Source: CAD feature listing. Evaluate the final solid. Frame: model axes, mm. A direction names the side the tool comes from. Give positions to 0.01 mm unless a question says otherwise; leave off trailing zeros. Order: outer loops, then holes, each group sorted by start corner. A loop starts at its lowest first (then second) coordinate and runs counter-clockwise, first axis right, second up. Notation, with made-up numbers: (76.5, 44) -> (133.5, 44) arc R16 ccw to (133.5, 74) -> close; hole circle Ø6 at (29.5, -8). An arc over 180 degrees is marked (long way). Answer in a Markdown table with one row per item.
```python
from build123d import *

# Parameters (mm, degrees)
F0_W         = 80
F0_H         = 60
F0_W_2       = 72
F0_H_2       = 52
F0_R         = 3
F0_R_2       = 2
F1_DEPTH     = 4
F2_DEPTH     = 30
F3_DEPTH     = 16
F5_R         = 12
F6_R         = 15
F7_S5_R      = 12
F7_T6_DEPTH  = 15
F7_S11_R     = 12
F7_T12_DEPTH = 15
F7_S17_R     = 12
F7_T18_DEPTH = 15
F7_S23_R     = 12
F7_T24_DEPTH = 15


# Not quite as in the source:
# - a fillet or chamfer that OpenCascade refuses, or shapes differently, is made with other operations: its cross-section is extruded or revolved along the edge and cut away or added


with BuildPart() as f1:
    # F0 (on Top) → F1 (new body)
    with BuildSketch(Plane.XY):
        Rectangle(F0_W, F0_H)
        Rectangle(F0_W_2, F0_H_2, mode=Mode.SUBTRACT)
        Rectangle(F0_W_2, F0_H_2)
        with Locations((-30, -20)):
            Circle(F0_R, mode=Mode.SUBTRACT)
        with Locations((30, -20)):
            Circle(F0_R, mode=Mode.SUBTRACT)
        with Locations((-30, 20)):
            Circle(F0_R, mode=Mode.SUBTRACT)
        with Locations((30, 20)):
            Circle(F0_R, mode=Mode.SUBTRACT)
        with Locations((-30, 20)):
            Circle(F0_R)
        with Locations((-30, 20)):
            Circle(F0_R_2, mode=Mode.SUBTRACT)
        with Locations((30, 20)):
            Circle(F0_R)
        with Locations((30, 20)):
            Circle(F0_R_2, mode=Mode.SUBTRACT)
        with Locations((30, -20)):
            Circle(F0_R)
        with Locations((30, -20)):
            Circle(F0_R_2, mode=Mode.SUBTRACT)
        with Locations((-30, -20)):
            Circle(F0_R)
        with Locations((-30, -20)):
            Circle(F0_R_2, mode=Mode.SUBTRACT)
    extrude(amount=F1_DEPTH)

    # F0 (on Top) → F2 (join)
    with BuildSketch(Plane.XY):
        Rectangle(F0_W, F0_H)
        Rectangle(F0_W_2, F0_H_2, mode=Mode.SUBTRACT)
    extrude(amount=F2_DEPTH)

    # F0 (on Top) → F3 (join)
    with BuildSketch(Plane.XY):
        with Locations((-30, 20)):
            Circle(F0_R)
        with Locations((-30, 20)):
            Circle(F0_R_2, mode=Mode.SUBTRACT)
        with Locations((-30, -20)):
            Circle(F0_R)
        with Locations((-30, -20)):
            Circle(F0_R_2, mode=Mode.SUBTRACT)
        with Locations((30, 20)):
            Circle(F0_R)
        with Locations((30, 20)):
            Circle(F0_R_2, mode=Mode.SUBTRACT)
        with Locations((30, -20)):
            Circle(F0_R)
        with Locations((30, -20)):
            Circle(F0_R_2, mode=Mode.SUBTRACT)
    extrude(amount=F3_DEPTH)

    # F4: union 

    # F5
    f5_edges = [f1.edges().sort_by_distance(p)[0] for p in [
        (-36, 26, 17),
        (36, 26, 17),
        (-36, -26, 17),
        (36, -26, 17),
    ]]
    fillet(f5_edges, radius=F5_R)

    # F6
    f6_edges = [f1.edges().sort_by_distance(p)[0] for p in [
        (40, -30, 15),
        (-40, -30, 15),
        (40, 30, 15),
        (-40, 30, 15),
    ]]
    fillet(f6_edges, radius=F6_R)

    # F7: fillet of radius 5.5 on 4 edges, made by hand


with BuildPart() as f7_tool2:
    # F7_s3 → F7_t4 (revolve)
    with BuildSketch(Plane.XZ.offset(-20)):
        with BuildLine():
            ThreePointArc((-21.4990343146, 3.9996), (-25.3890872965, 5.6109127035), (-27.0004, 9.5009656854))
            Line((-27.0004, 9.5009656854), (-27.5505365685, 9.5009656854))
            ThreePointArc((-27.5505365685, 9.5009656854), (-27.5501365685, 6.7504828427), (-27.5501365685, 4))
            Line((-27.5501365685, 4), (-27, 3.4498634315))
            ThreePointArc((-27, 3.4498634315), (-24.2495171573, 3.4498634315), (-21.4990343146, 3.4494634315))
            Line((-21.4990343146, 3.4494634315), (-21.4990343146, 3.9996))
        make_face()
    revolve(axis=Axis((-30, 20, 4), (0, 0, -1)))

    # F7_s5 → F7_t6 (intersect, symmetric)
    with BuildSketch(Plane.XY.offset(8.4)):
        with Locations((-24, 14)):
            Circle(F7_S5_R)
    extrude(amount=F7_T6_DEPTH, both=True, mode=Mode.INTERSECT)


with BuildPart() as f1_1:
    add(f1.part)

    # F7_t1: union F7_tool2
    add(f7_tool2.part)


with BuildPart() as f7_tool8:
    # F7_s9 → F7_t10 (revolve)
    with BuildSketch(Plane.XZ.offset(20)):
        with BuildLine():
            ThreePointArc((-21.4990343146, 3.9996), (-25.3890872965, 5.6109127035), (-27.0004, 9.5009656854))
            Line((-27.0004, 9.5009656854), (-27.5505365685, 9.5009656854))
            ThreePointArc((-27.5505365685, 9.5009656854), (-27.5501365685, 6.7504828427), (-27.5501365685, 4))
            Line((-27.5501365685, 4), (-27, 3.4498634315))
            ThreePointArc((-27, 3.4498634315), (-24.2495171573, 3.4498634315), (-21.4990343146, 3.4494634315))
            Line((-21.4990343146, 3.4494634315), (-21.4990343146, 3.9996))
        make_face()
    revolve(axis=Axis((-30, -20, 4), (0, 0, -1)))

    # F7_s11 → F7_t12 (intersect, symmetric)
    with BuildSketch(Plane.XY.offset(8.4)):
        with Locations((-24, -14)):
            Circle(F7_S11_R)
    extrude(amount=F7_T12_DEPTH, both=True, mode=Mode.INTERSECT)


with BuildPart() as f1_2:
    add(f1_1.part)

    # F7_t7: union F7_tool8
    add(f7_tool8.part)


with BuildPart() as f7_tool14:
    # F7_s15 → F7_t16 (revolve)
    with BuildSketch(Plane.XZ.offset(-20)):
        with BuildLine():
            ThreePointArc((38.5009656854, 3.9996), (34.6109127035, 5.6109127035), (32.9996, 9.5009656854))
            Line((32.9996, 9.5009656854), (32.4494634315, 9.5009656854))
            ThreePointArc((32.4494634315, 9.5009656854), (32.4498634315, 6.7504828427), (32.4498634315, 4))
            Line((32.4498634315, 4), (33, 3.4498634315))
            ThreePointArc((33, 3.4498634315), (35.7504828427, 3.4498634315), (38.5009656854, 3.4494634315))
            Line((38.5009656854, 3.4494634315), (38.5009656854, 3.9996))
        make_face()
    revolve(axis=Axis((30, 20, 4), (0, 0, -1)))

    # F7_s17 → F7_t18 (intersect, symmetric)
    with BuildSketch(Plane.XY.offset(8.4)):
        with Locations((24, 14)):
            Circle(F7_S17_R)
    extrude(amount=F7_T18_DEPTH, both=True, mode=Mode.INTERSECT)


with BuildPart() as f1_3:
    add(f1_2.part)

    # F7_t13: union F7_tool14
    add(f7_tool14.part)


with BuildPart() as f7_tool20:
    # F7_s21 → F7_t22 (revolve)
    with BuildSketch(Plane.XZ.offset(20)):
        with BuildLine():
            ThreePointArc((38.5009656854, 3.9996), (34.6109127035, 5.6109127035), (32.9996, 9.5009656854))
            Line((32.9996, 9.5009656854), (32.4494634315, 9.5009656854))
            ThreePointArc((32.4494634315, 9.5009656854), (32.4498634315, 6.7504828427), (32.4498634315, 4))
            Line((32.4498634315, 4), (33, 3.4498634315))
            ThreePointArc((33, 3.4498634315), (35.7504828427, 3.4498634315), (38.5009656854, 3.4494634315))
            Line((38.5009656854, 3.4494634315), (38.5009656854, 3.9996))
        make_face()
    revolve(axis=Axis((30, -20, 4), (0, 0, -1)))

    # F7_s23 → F7_t24 (intersect, symmetric)
    with BuildSketch(Plane.XY.offset(8.4)):
        with Locations((24, -14)):
            Circle(F7_S23_R)
    extrude(amount=F7_T24_DEPTH, both=True, mode=Mode.INTERSECT)


with BuildPart() as f1_4:
    add(f1_3.part)

    # F7_t19: union F7_tool20
    add(f7_tool20.part)


solid = f1_4.part
```
(1) Pull-direction query (X, two-part tool) for faces 3 (the cylindrical face through (-28.092, -19.399, 7.888)), 4 (the cylindrical face through (-32.58, -22.39, 17.18)), 5 (the flat face through (-40, 0, 15)), 6 (the cylindrical face through (35.49, 25.72, 14.79)); classes: +X half, -X half, draft (parallel to the pull), parting line (faces both ways), or undercut.
A:
| item | result |
|---|---|
| face 3 | undercut |
| face 4 | undercut |
| face 5 | -X half |
| face 6 | +X half |
(2) First-contact query: pin 1 Ø2.5 at (x, y) = (30, 20) entering from +Z; pin 2 Ø5 at (x, y) = (-31, -19.5) entering from +Z; pin 3 Ø15.5 at (x, y) = (-15, 9) entering from +Z; pin 4 Ø3 at (x, y) = (-23, 16) entering from +Z. Flat tips, straight axial feed; report the tip coordinate or a pass-through.
A:
| item | result |
|---|---|
| pin 1 | passes through |
| pin 2 | stops at z = 16 |
| pin 3 | stops at z = 4 |
| pin 4 | stops at z = 4.35 |
(3) Section query C-C (z = 18). Return the cut outline in (x, y).
A:
| item | result |
|---|---|
| outline | (-40, -15) arc R15 ccw to (-25, -30) -> (25, -30) arc R15 ccw to (40, -15) -> (40, 15) arc R15 ccw to (25, 30) -> (-25, 30) arc R15 ccw to (-40, 15) -> close; hole (-36, -14) arc R12 ccw to (-24, -26) -> (24, -26) arc R12 ccw to (36, -14) -> (36, 14) arc R12 ccw to (24, 26) -> (-24, 26) arc R12 ccw to (-36, 14) -> close |
(4) Section query A-A (z = 13). Give the number of separate pieces and of enclosed holes in the cut face, plus the area to 3 significant figures.
A:
| item | result |
|---|---|
| separate pieces | 5 |
| enclosed holes | 5 |
| area | 1,050 mm^2 |
(5) Section query D-D (y = -3). Return the cut outline in (x, z).
A:
| item | result |
|---|---|
| outline | (-40, 0) -> (40, 0) -> (40, 30) -> (36, 30) -> (36, 4) -> (-36, 4) -> (-36, 30) -> (-40, 30) -> close |
(6) Section query B-B (x = -18). Return the cut outline in (y, z), plus the area to 3 significant figures.
A:
| item | result |
|---|---|
| outline | (-30, 0) -> (30, 0) -> (30, 30) -> (26, 30) -> (26, 4) -> (-26, 4) -> (-26, 30) -> (-30, 30) -> close |
| area | 448 mm^2 |
(7) Access query for faces 1 (the cylindrical face through (-33, -20, 13)), 2 (the cylindrical face through (35.49, -25.72, 15.21)). Directions: +Z, -Z, +X, -X, +Y, -Y. A direction counts if a zero-diameter tool reaches every point of the face in a straight line with its end or side. Return the directions, or none.
A:
| item | result |
|---|---|
| face 1 | +Z |
| face 2 | +Z, -Z, +X, -Y |
(8) Ray query, probe 1 along X at (y, z) = (-2, 8.5); probe 2 along Y at (x, z) = (12, 24); probe 3 along X at (y, z) = (19, 7.5). Return the intervals inside material, ascending.
A:
| item | result |
|---|---|
| probe 1 | x = -40 to -36, 36 to 40 |
| probe 2 | y = -30 to -26, 26 to 30 |
| probe 3 | x = -39.46 to -34.91, -33.22 to -31.73, -28.27 to -26.78, 26.78 to 28.27, 31.73 to 33.22, 34.91 to 39.46 |
